```python
from build123d import *

# Parameters (mm, degrees)
SKETCH_1_R          = 2.7
SKETCH_1_R_2        = 2.5
SKETCH_1_R_3        = 3.5
EXTRUDE_1_DEPTH     = 4
SKETCH_2_R          = 6.01
CUT_EXTRUDE_1_DEPTH = 1
SKETCH_3_R          = 6.01
CUT_EXTRUDE_2_DEPTH = 1
CUT_EXTRUDE_START   = -1
SKETCH_4_R          = 6.01
CUT_EXTRUDE_3_DEPTH = 1
SKETCH_5_R          = 4.505
CUT_EXTRUDE_4_DEPTH = 137.097733658
FILLET_1_R          = 10


with BuildPart() as part:
    # 草图1 → 凸台-拉伸1 (new body)
    with BuildSketch(Plane(origin=(0, 0, 0), x_dir=(1, 0, 0), z_dir=(0, 1, 0))):
        with BuildLine():
            Line((4.358898944, -9), (121.312001056, -9))
            ThreePointArc((121.312001056, -9), (135.6709, 0), (121.312001056, 9))
            Line((121.312001056, 9), (4.358898944, 9))
            ThreePointArc((4.358898944, 9), (-10, 0), (4.358898944, -9))
        make_face()
        with Locations(Location((0, 0, 0), (0, 0, 270))):
            Circle(SKETCH_1_R, mode=Mode.SUBTRACT)
        with Locations(Location((125.6709, 0, 0), (0, 0, 270))):
            Circle(SKETCH_1_R_2, mode=Mode.SUBTRACT)
        with Locations(Location((62.83545, 0, 0), (0, 0, 270))):
            Circle(SKETCH_1_R_3, mode=Mode.SUBTRACT)
        with BuildLine():
            Line((49.395542126, -3.5), (14.395542126, -3.5))
            ThreePointArc((14.395542126, -3.5), (10.895542126, 0), (14.395542126, 3.5))
            Line((14.395542126, 3.5), (49.395542126, 3.5))
            ThreePointArc((49.395542126, 3.5), (52.895542126, 0), (49.395542126, -3.5))
        make_face(mode=Mode.SUBTRACT)
        with BuildLine():
            Line((76.275357874, -3.5), (111.275357874, -3.5))
            ThreePointArc((111.275357874, -3.5), (114.775357874, 0), (111.275357874, 3.5))
            Line((111.275357874, 3.5), (76.275357874, 3.5))
            ThreePointArc((76.275357874, 3.5), (72.775357874, 0), (76.275357874, -3.5))
        make_face(mode=Mode.SUBTRACT)
    extrude(amount=EXTRUDE_1_DEPTH)

    # 草图2 → 切除-拉伸1 (cut)
    with BuildSketch(Plane.XZ):
        with Locations(Location((125.6709, 0, 0), (0, 0, 270))):
            Circle(SKETCH_2_R)
    extrude(amount=-CUT_EXTRUDE_1_DEPTH, mode=Mode.SUBTRACT)

    # 草图3 → 切除-拉伸2 (cut)
    with BuildSketch(Plane(origin=(0, 4, 0), x_dir=(1, 0, 0), z_dir=(0, 1, 0))):
        with Locations(Location((0, 0, 0), (0, 0, 270))):
            Circle(SKETCH_3_R)
    extrude(amount=-CUT_EXTRUDE_2_DEPTH, mode=Mode.SUBTRACT)

    # 草图4 → 切除-拉伸3 (cut)
    with BuildSketch(Plane.XZ.offset(CUT_EXTRUDE_START)):
        with Locations(Location((0, 0, 0), (0, 0, 90))):
            Circle(SKETCH_4_R)
    extrude(amount=CUT_EXTRUDE_3_DEPTH, mode=Mode.SUBTRACT)

    # 草图5 → 切除-拉伸4 (cut, through all)
    with BuildSketch(Plane(origin=(0, 4, 0), x_dir=(1, 0, 0), z_dir=(0, 1, 0))):
        with Locations(Location((125.6709, 0, 0), (0, 0, 270))):
            Circle(SKETCH_5_R)
    extrude(amount=-CUT_EXTRUDE_4_DEPTH, mode=Mode.SUBTRACT)

    # 圆角1
    fillet_1_edges = [part.edges().sort_by_distance(p)[0] for p in [
        (4.358898944, 2, -9),
        (121.312001056, 2, -9),
        (121.312001056, 2, 9),
        (4.358898944, 2, 9),
    ]]
    fillet(fillet_1_edges, radius=FILLET_1_R)


solid = part.part
```
Source: CAD feature listing. Evaluate the final solid. Frame: model axes, mm. A direction names the side the tool comes from. Coordinates: 2 decimals unless noted, no trailing zeros. Order: outer loops, then holes, each group sorted by start corner. A loop starts at its lowest first (then second) coordinate and runs counter-clockwise, first axis right, second up. Notation, with made-up numbers: M -34,70 L -6,70 A30 ccw -6,96 Z; hole C 37,0.5 d8. An arc over 180 degrees is marked long. Write each question's results on one line, items separated by ' | '. Start each with the question number.
1) Contact query for flat-ended pins moving along their axis: pin 1 Ø2 at (x, y) = (99.5, 2) entering from +Z; pin 2 Ø1 at (y, z) = (1, 1) entering from -X; pin 3 Ø11 at (x, z) = (0, 0) entering from -Y; pin 4 Ø5.5 at (x, z) = (125.67, 0) entering from +Y. Output: stop coordinate, or through.
2) Section query A-A (x = 0). Return the cut outline in (y, z).
3) Section query D-D (x = 24.5). Return the cut outline in (y, z), plus the area to 3 significant figures.
4) Access query for faces 1 (the face through (121, 1, 1)), 2 (the face through (32, 2, -3.5)), 3 (the face through (-3, 3, 1)). Directions: +Z, -Z, +X, -X, +Y, -Y. A direction counts if a zero-diameter tool reaches every point of the face in a straight line with its end or side. Return the directions, or none.
5) Line query: line 1 (X direction, y = 1.95, z = 0); line 2 (X direction, y = 0.2, z = 0); line 3 (Z direction, x = 25, y = 2.2). Output: solid intervals per line, ascending. Write a range as from..to.
6) Section query C-C (y = 1.7). Return the cut outline in (x, z) (1 decimal).
7) Draft query along Z for faces 4 (the face through (131.63, 0.49, 0.78)), 5 (the face through (62, 2, 9)), 6 (the face through (64, 2, -9)), 7 (the face through (94, 2, 3.5)). Return one class per face: released by +Z, released by -Z, zero draft, split by the parting line, or undercut.
8) Section query B-B (z = 0). Give the number of separate pieces and of enclosed holes in the cut face, plus the area to 3 significant figures.
Answers:
1) pin 1: stops at z = 9 | pin 2: stops at x = -9.99 | pin 3: stops at y = 1 | pin 4: passes through
2) outline: M 0,-10 L 4,-10 L 4,-6.01 L 3,-6.01 L 3,-2.7 L 1,-2.7 L 1,-6.01 L 0,-6.01 Z; M 0,6.01 L 1,6.01 L 1,2.7 L 3,2.7 L 3,6.01 L 4,6.01 L 4,10 L 0,10 Z
3) outline: M 0,-9 L 4,-9 L 4,-3.5 L 0,-3.5 Z; M 0,3.5 L 4,3.5 L 4,9 L 0,9 Z | area: 44.0 mm^2
4) face 1: -Y | face 2: +Y, -Y | face 3: +Y
5) line 1: x = -10..-2.7, 2.7..10.9, 52.9..59.34, 66.34..72.78, 114.78..121.17, 130.18..135.67 | line 2: x = -10..-6.01, 6.01..10.9, 52.9..59.34, 66.34..72.78, 114.78..119.66, 131.68..135.67 | line 3: z = -9..-3.5, 3.5..9
6) outline: M 3.1,-9.5 A10 cw 6.2,-9 L 119.4,-9 A10 cw 122.5,-9.5 A10 ccw long 122.5,9.5 A10 cw 119.4,9 L 6.2,9 A10 cw 3.1,9.5 A10 ccw long Z; hole C 0,0 d5.4; hole M 14.4,-3.5 L 49.4,-3.5 A3.5 ccw 49.4,3.5 L 14.4,3.5 A3.5 ccw Z; hole C 62.8,0 d7; hole M 76.3,-3.5 L 111.3,-3.5 A3.5 ccw 111.3,3.5 L 76.3,3.5 A3.5 ccw Z; hole C 125.7,0 d9
7) face 4: undercut | face 5: released by +Z | face 6: released by -Z | face 7: undercut
8) separate pieces: 6 | enclosed holes: 0 | area: 145 mm^2
